Can you work these out from the drawing? Everything is in mm from the part's minimum corner. A direction names the side the tool comes from. Coordinates: 2 decimals unless noted, no trailing zeros. Write each loop counter-clockwise with the first axis right and the second up, starting at its lowest first coordinate (ties: lowest second). Pieces come first, ordered by that corner, then holes. Notation, with made-up numbers: M 44,8 L 68,8 A12 ccw 68,19 Z; hole C 48.25,47.25 d9. An arc over 180 degrees is marked long. Use one line per item in the form item = value. Start each with the question number.
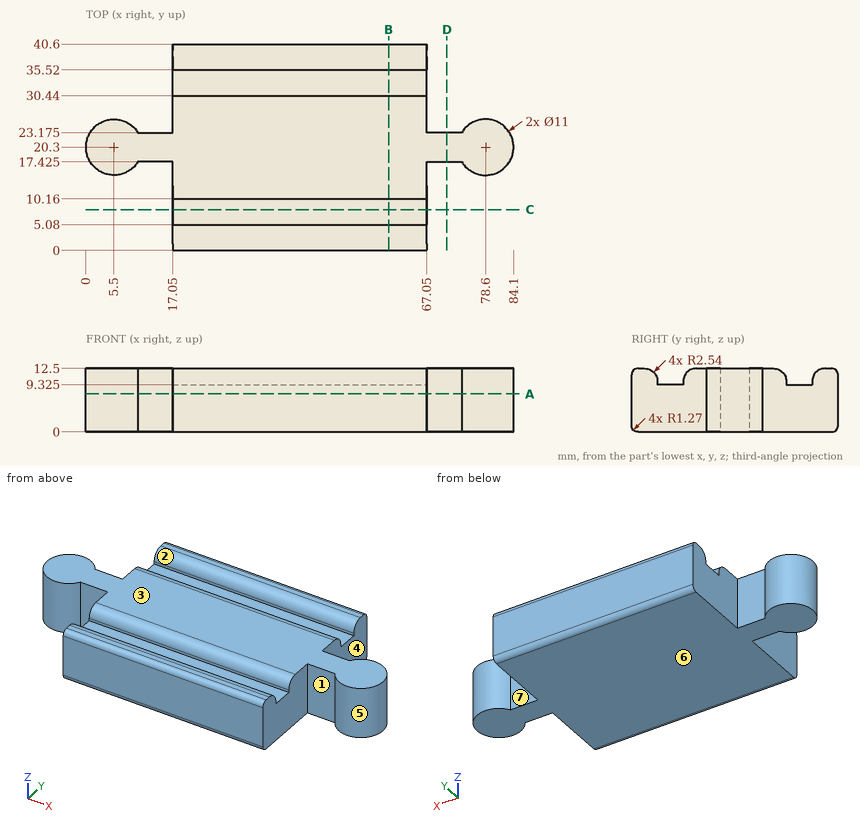
1) Please list where these lines run through material, in increasing order: line 1 (Y direction, x = 46.5, z = 9.5); line 2 (Y direction, x = 67, z = 11.25); line 3 (Y direction, x = 71, z = 9.25) (3 decimals).
2) Suppose I cut it at C-C on y = 8. Please give me the cut outline in (x, z) (3 decimals).
3) If we mould it in two halves opening along X, with no side actions, what happens to the marked faces 6 and 7? For each: +X half, -X half, draft (parallel to the pull), parting line (faces both ways), or undercut.
4) Which directions (+Z, -Z, +X, -X, +Y, -Y) give clear straight access to the entire face, cutting with the end or side of a thin tool? Please do the marked faces 1, 2, 3, 4 and 5.
5) Suppose I cut it at B-B on x = 59.5. Please give me the cut outline in (y, z) (3 decimals), and give its area (3 significant figures).
6) Will these pins go through, and if not, where does the flat tip stop? pin 1 Ø6 at (x, z) = (64, 5.5) entering from -Y; pin 2 Ø3 at (y, z) = (34, 8) entering from +X; pin 3 Ø5.5 at (x, y) = (38.5, 7.5) entering from +Z; pin 4 Ø5 at (x, y) = (47, 6) entering from +Z.
7) Suppose I cut it at D-D on x = 71. Please give me the cut outline in (y, z) (3 decimals).
8) Suppose I cut it at A-A on z = 7.5. Please give me the cut outline in (x, y) (3 decimals).
Computed values:
q1.line_1 = 0 to 5.08, 10.16 to 30.44, 35.52 to 40.6
q1.line_2 = 0 to 4.73, 10.51 to 30.09, 35.87 to 40.6
q1.line_3 = 17.425 to 23.175
q2.outline = M 17.05,0 L 67.05,0 L 67.05,9.325 L 17.05,9.325 Z
q3.face_6 = draft
q3.face_7 = undercut
q4.face_1 = +Z, -Z, -Y
q4.face_2 = +Z, +X, -X
q4.face_3 = +Z, +X, -X, +Y, -Y
q4.face_4 = +Z, -Z, +Y
q4.face_5 = +Z, -Z
q5.outline = M 0,1.27 A1.27 ccw 1.27,0 L 39.33,0 A1.27 ccw 40.6,1.27 L 40.6,11.23 A1.27 ccw 39.33,12.5 L 38.06,12.5 A2.54 ccw 35.52,9.96 L 35.52,9.325 L 30.44,9.325 L 30.44,9.96 A2.54 ccw 27.9,12.5 L 12.7,12.5 A2.54 ccw 10.16,9.96 L 10.16,9.325 L 5.08,9.325 L 5.08,9.96 A2.54 ccw 2.54,12.5 L 1.27,12.5 A1.27 ccw 0,11.23 Z
q5.area = 468 mm²
q6.pin_1 = 0
q6.pin_2 = 67.05
q6.pin_3 = 11.21
q6.pin_4 = 12.31
q7.outline = M 17.425,0 L 23.175,0 L 23.175,12.5 L 17.425,12.5 Z
q8.outline = M 10.189,17.425 L 17.05,17.425 L 17.05,0 L 67.05,0 L 67.05,17.425 L 73.911,17.425 A5.5 ccw long 73.911,23.175 L 67.05,23.175 L 67.05,40.6 L 17.05,40.6 L 17.05,23.175 L 10.189,23.175 A5.5 ccw long Z
